from build123d import *

# Parameters (mm, degrees)
PAD_DEPTH         = 4
SKETCH001_W       = 30
SKETCH001_H       = 58.56
PAD001_DEPTH      = 8.65
SKETCH002_R       = 1.58
PAD002_DEPTH      = 6
SKETCH003_R       = 1.58
POCKET_DEPTH      = 4.651
POCKET_DEPTH_BACK = 22.255879


with BuildPart() as key:
    # Sketch → Pad (new body)
    with BuildSketch(Plane.XY):
        with BuildLine():
            Line((-3.78, 0), (-3.78, 36))
            Line((-3.78, 36), (-4.11555, 36))
            ThreePointArc((-4.11555, 43.56), (-7.89555, 39.78), (-4.11555, 36))
            Line((-4.11555, 43.56), (4.11555, 43.56))
            ThreePointArc((4.11555, 36), (7.89555, 39.78), (4.11555, 43.56))
            Line((3.78, 36), (4.11555, 36))
            Line((3.78, 0), (3.78, 36))
            Line((-3.78, 0), (3.78, 0))
        make_face()
    pad = extrude(amount=PAD_DEPTH)

    # Mirrored: Pad across Sketch H_Axis
    add(pad.mirror(Plane.ZX))


with BuildPart() as cut:
    # Sketch001 → Pad001 (new body)
    with BuildSketch(Plane.XY.offset(-4.65)):
        with Locations((0, -29.28)):
            Rectangle(SKETCH001_W, SKETCH001_H)
    extrude(amount=PAD001_DEPTH)

    # Sketch002 → Pad002 (join)
    with BuildSketch(Plane.XZ.offset(58.56)):
        with BuildLine():
            ThreePointArc((26.5, 0), (0, 22.254879), (-26.5, 0))
            Line((-26.5, -2.325), (-26.5, 0))
            Line((-26.5, -4.65), (-26.5, -2.325))
            Line((-26.5, -4.65), (26.5, -4.65))
            Line((26.5, 0), (26.5, -4.65))
        make_face()
        with Locations((-19.403194, 6.552439)):
            Circle(SKETCH002_R, mode=Mode.SUBTRACT)
        with Locations((19.403194, 6.552439)):
            Circle(SKETCH002_R, mode=Mode.SUBTRACT)
        with Locations((0, 17.754879)):
            Circle(SKETCH002_R, mode=Mode.SUBTRACT)
        with Locations((0, 11.854879)):
            Circle(SKETCH002_R, mode=Mode.SUBTRACT)
    extrude(amount=-PAD002_DEPTH)

    # Sketch003 → Pocket (cut, two sides)
    with BuildSketch(Plane.XY) as pocket_sk:
        with Locations((-4.11555, -39.78)):
            Circle(SKETCH003_R)
        with Locations((4.11555, -39.78)):
            Circle(SKETCH003_R)
    extrude(amount=-POCKET_DEPTH, mode=Mode.SUBTRACT)
    extrude(pocket_sk.sketch, amount=POCKET_DEPTH_BACK, mode=Mode.SUBTRACT)

    # Cut: cut key
    add(key.part, mode=Mode.SUBTRACT)


solid = cut.part
Design review of the part built by this model. Coordinates are the model's own, in mm. A direction names the side the tool comes from. Coordinates: 2 decimals unless noted, no trailing zeros. Order: outer loops, then holes, each group sorted by start corner. A loop starts at its lowest first (then second) coordinate and runs counter-clockwise, first axis right, second up.
Item 1: For faces 4 (the flat face through (-3.78, -18, 2)), 5 (the cylindrical face through (-7.895, -39.863, 1.972)), 6 (the flat face through (-7, -26, 4)), 7 (the flat face through (15, -27, 0)), list the 3-axis set-ups (+Z, -Z, +X, -X, +Y, -Y) from which the entire face can be reached by the end or side of a thin tool; tool diameter is ignored.
Item 2: Take a section at D-D, the plane y = -23. Write out the cut boundary in (x, z).
Item 3: Take a section at C-C, the plane z = -2. Write out the cut boundary in (x, y), then the cut area to 3 significant figures.
Item 4: For pin 1 Ø1.9 at (x, z) = (0, 11.85) entering from -Y; pin 2 Ø3 at (y, z) = (-24, 1) entering from +X; pin 3 Ø3.5 at (x, z) = (19.4, 6.55) entering from +Y; pin 4 Ø2 at (x, z) = (1.5, 2.5) entering from +Y, all flat-tipped, find the tip position at first contact; note any pin that passes through.
Item 5: The part is to be moulded in two halves that separate along X. For faces 1 (the cylindrical face through (-4.321, -38.213, -2.292)), 2 (the flat face through (0, -58.56, 6)), 3 (the flat face through (26.5, -56, -2)), say which applies: pulls with the +X half, pulls with the -X half, needs draft (parallel to the pull), parting line crosses it, or undercut.
Item 6: Take a section at A-A, the plane x = 0. Write out the cut boundary in (y, z), then the cut area to 3 significant figures.
Item 7: Take a section at B-B, the plane y = -39.78. Write out the cut boundary in (x, z), then the cut area to 3 significant figures.
Item 8: For line 1 (X direction, y = -8, z = 2.5); line 2 (Y direction, x = -5, z = 11.5); line 3 (Z direction, x = -12.5, y = -23), list the stretches that pass through material, from the lowest coordinate up.
The answers:
1. face 4: +Z, +Y
1. face 5: +Z
1. face 6: +Z, +X, -X, +Y
1. face 7: +Z, -Z, +X, +Y
2. outline: (-15, -4.65) - (15, -4.65) - (15, 4) - (3.78, 4) - (3.78, 0) - (-3.78, 0) - (-3.78, 4) - (-15, 4) - close
3. outline: (-26.5, -58.56) - (26.5, -58.56) - (26.5, -52.56) - (15, -52.56) - (15, 0) - (-15, 0) - (-15, -52.56) - (-26.5, -52.56) - close; hole circle Ø3.16 at (-4.12, -39.78); hole circle Ø3.16 at (4.12, -39.78)
3. area: 1,880 mm2
4. pin 1: passes through
4. pin 2: stops at x = 15
4. pin 3: stops at y = -52.56
4. pin 4: stops at y = -43.56
5. face 1: undercut
5. face 2: needs draft
5. face 3: pulls with the +X half
6. outline: (-58.56, -4.65) - (0, -4.65) - (0, 0) - (-43.56, 0) - (-43.56, 4) - (-52.56, 4) - (-52.56, 10.27) - (-58.56, 10.27) - close; (-58.56, 13.43) - (-52.56, 13.43) - (-52.56, 16.17) - (-58.56, 16.17) - close; (-58.56, 19.33) - (-52.56, 19.33) - (-52.56, 22.25) - (-58.56, 22.25) - close
6. area: 404 mm2
7. outline: (-15, -4.65) - (-5.7, -4.65) - (-5.7, 0) - (-7.9, 0) - (-7.9, 4) - (-15, 4) - close; (-2.54, -4.65) - (2.54, -4.65) - (2.54, 0) - (-2.54, 0) - close; (5.7, -4.65) - (15, -4.65) - (15, 4) - (7.9, 4) - (7.9, 0) - (5.7, 0) - close
7. area: 167 mm2
8. line 1: x = -15 to -3.78, 3.78 to 15
8. line 2: y = -58.56 to -52.56
8. line 3: z = -4.65 to 4
